from build123d import *

# Parameters (mm, degrees)
SKETCH_1_W                   = 26
SKETCH_1_H                   = 15
EXTRUDE_1_DEPTH              = 3
EXTRUDE_2_DEPTH              = 15
HOLE_WIZARD_M5_2_D           = 4.2
HOLE_WIZARD_M5_2_DEPTH       = 12.4
HOLE_WIZARD_M5_2_CSINK_D     = 5.05
HOLE_WIZARD_M5_2_CSINK_ANGLE = 90
HOLE_WIZARD_M5_2_TIP         = 1.2618073


with BuildPart() as part:
    # 草图1 → 凸台-拉伸1 (new body)
    with BuildSketch(Plane(origin=(0, 0, 0), x_dir=(1, 0, 0), z_dir=(0, 1, 0))):
        with Locations((13, 7.5)):
            Rectangle(SKETCH_1_W, SKETCH_1_H)
    extrude(amount=EXTRUDE_1_DEPTH)

    # 草图3 → 凸台-拉伸2 (add)
    with BuildSketch(Plane.XY):
        with BuildLine():
            Line((9.001058493, 3), (11.575219315, 3))
            ThreePointArc((11.575219315, 3), (5.300234972, 6.410185465), (2.8, 13.1))
            Line((2.8, 13.1), (2.137148939, 13.1))
            ThreePointArc((2.137148939, 13.1), (4.015528976, 6.994198366), (9.001058493, 3))
        make_face()
        with BuildLine():
            Line((23.2, 13.1), (23.862851061, 13.1))
            ThreePointArc((23.862851061, 13.1), (21.984471024, 6.994198366), (16.998941507, 3))
            Line((16.998941507, 3), (14.424780685, 3))
            ThreePointArc((14.424780685, 3), (20.699765028, 6.410185465), (23.2, 13.1))
        make_face()
    extrude(amount=-EXTRUDE_2_DEPTH)

    # M5 螺纹孔2
    with Locations(Plane.XZ):
        with Locations((7, -7.5), (19, -7.5)):
            CounterSinkHole(HOLE_WIZARD_M5_2_D / 2, HOLE_WIZARD_M5_2_CSINK_D / 2, depth=HOLE_WIZARD_M5_2_DEPTH, counter_sink_angle=HOLE_WIZARD_M5_2_CSINK_ANGLE)
            with Locations((0, 0, -(HOLE_WIZARD_M5_2_DEPTH + HOLE_WIZARD_M5_2_TIP / 2))):  # 118° drill point
                Cone(0, HOLE_WIZARD_M5_2_D / 2, HOLE_WIZARD_M5_2_TIP, mode=Mode.SUBTRACT)


solid = part.part
Could you check a few things on this model? Use its own coordinates, in mm. A direction names the side the tool comes from. Round coordinates to 2 decimals unless told otherwise and drop trailing zeros. Write each loop counter-clockwise with the first axis right and the second up, starting at its lowest first coordinate (ties: lowest second). Pieces come first, ordered by that corner, then holes. Notation, with made-up numbers: (-18.5, -9.5) - (-14.5, -9.5) arc R19 cw to (-14.5, -1.5) - close; hole circle Ø8 at (-1.75, 74). An arc over 180 degrees is marked (long way). Put each result on its own line as item: value. Start each with the question number.
(1) Thinking about a two-plate mould opening in Z: for faces 1 (the cylindrical face through (20.666, 2.269, -8.778)), 2 (the flat face through (12.9, 2.6, -15)), 3 (the flat face through (26, 1, -7)), which applies, released by +Z, released by -Z, zero draft, split by the parting line, or undercut?
(2) I want a section at D-D, the plane y = 4.25. Please give me the cut outline in (x, z).
(3) I want a section at C-C, the plane x = 19. Please give me the cut outline in (y, z) (3 decimals), plus the area to 3 significant figures.
(4) I need wall thicknesses on probe 1 along Z at (x, y) = (7, 2.5); probe 2 along X at (y, z) = (7.5, -3.5); probe 3 along Y at (x, z) = (13.5, -12.75). Which ranges of each line are inside material? Lowest first, please.
(5) I want a section at B-B, the plane z = -7.5. Please give me the cut outline in (x, y) (3 decimals).
(6) Will these pins go through, and if not, where does the flat tip stop? pin 1 (5 mm diameter, centred on y = 9.5, z = -7, fed in from -X); pin 2 (5 mm diameter, centred on x = 14, z = -11, fed in from -Y); pin 3 (1.4 mm diameter, centred on x = 13.5, z = -4.5, fed in from +Y); pin 4 (1 mm diameter, centred on y = 8.5, z = -4.5, fed in from +X).
(7) I want a section at A-A, the plane y = 7.25. Please give me the cut outline in (x, z).
(8) For faces 4 (the flat face through (12.9, 2.6, 0)), 5 (the flat face through (13, 3, -8)), which set-ups out of +Z, -Z, +X, -X, +Y, -Y let a thin tool reach every point of the face, with its end or its side?
Here are the results:
1. face 1: undercut
1. face 2: released by -Z
1. face 3: zero draft
2. outline: (6.7, -15) - (7.93, -15) - (7.93, -9.38) arc R2.1 cw to (6.7, -9.58) - close; (6.7, -5.42) arc R2.1 cw to (7.93, -5.62) - (7.93, 0) - (6.7, 0) - close; (18.07, -15) - (19.3, -15) - (19.3, -9.58) arc R2.1 cw to (18.07, -9.38) - close; (18.07, -5.62) arc R2.1 cw to (19.3, -5.42) - (19.3, 0) - (18.07, 0) - close
3. outline: (0, -15) - (3, -15) - (3, -9.6) - (0.425, -9.6) - (0, -10.025) - close; (0, -4.975) - (0.425, -5.4) - (3, -5.4) - (3, 0) - (0, 0) - close; (4.045, -15) - (4.851, -15) - (4.851, -9.6) - (4.045, -9.6) - close; (4.045, -5.4) - (4.851, -5.4) - (4.851, 0) - (4.045, 0) - close
3. area: 40.9 mm^2
4. probe 1: z = -15 to -9.6, -5.4 to 0
4. probe 2: x = 3.69 to 4.47, 21.53 to 22.31
4. probe 3: y = 0 to 3
5. outline: (0, 0) - (4.475, 0) - (4.9, 0.425) - (4.9, 3) - (0, 3) - close; (2.137, 13.1) arc R10.863 ccw to (4.9, 5.862) - (4.9, 6.901) arc R10.2 cw to (2.8, 13.1) - close; (9.1, 0.425) - (9.525, 0) - (16.475, 0) - (16.9, 0.425) - (16.9, 3.675) arc R10.2 cw to (14.425, 3) - (11.575, 3) arc R10.2 cw to (9.1, 3.675) - close; (21.1, 0.425) - (21.525, 0) - (26, 0) - (26, 3) - (21.1, 3) - close; (21.1, 5.862) arc R10.863 ccw to (23.863, 13.1) - (23.2, 13.1) arc R10.2 cw to (21.1, 6.901) - close
6. pin 1: stops at x = 2.19
6. pin 2: stops at y = 0
6. pin 3: stops at y = 3
6. pin 4: stops at x = 23.06
7. outline: (3.85, -15) - (4.64, -15) - (4.64, 0) - (3.85, 0) - close; (21.36, -15) - (22.15, -15) - (22.15, 0) - (21.36, 0) - close
8. face 4: +Z, +X, -X, +Y, -Y
8. face 5: +Z, -Z, +Y
